Part model, mm, in its own coordinate system. Face numbers are marked on the shaded views. A direction names the side the tool comes from. Give positions to 0.01 mm unless a question says otherwise; leave off trailing zeros. Order: outer loops, then holes, each group sorted by start corner. A loop starts at its lowest first (then second) coordinate and runs counter-clockwise, first axis right, second up. Notation, with made-up numbers: (0.25, 69) - (23.25, 69) arc R28 cw to (23.25, 93) - close; hole circle Ø7 at (10.5, -18.5). An arc over 180 degrees is marked (long way). One line per item, written item: value.
```python
from build123d import *

# Parameters (mm, degrees)
F0_W     = 31.8262
F0_H     = 7.8232
F1_DEPTH = 9.6012
F3_R     = 2.4511
F4_DEPTH = 1.8288
F5_W     = 28.9814
F5_H     = 4.826
F6_DEPTH = 8.382
F7_R     = 1.4478
F8_DEPTH = 8.382


with BuildPart() as f1:
    # F0 (on Top) → F1 (new body)
    with BuildSketch(Plane.XY):
        Rectangle(F0_W, F0_H)
    extrude(amount=F1_DEPTH)

    # F3 (on face) → F4 (join)
    with BuildSketch(Plane.XY.offset(9.6012)):
        with Locations((11.9888, 0)):
            Circle(F3_R)
        with Locations((3.9116, 0)):
            Circle(F3_R)
        with Locations((-3.9116, 0)):
            Circle(F3_R)
        with Locations((-11.9888, 0)):
            Circle(F3_R)
    extrude(amount=F4_DEPTH)

    # F5 (on face) → F6 (cut)
    with BuildSketch(Plane(origin=(0, 0, 0), x_dir=(1, 0, 0), z_dir=(0, 0, -1))):
        Rectangle(F5_W, F5_H)
    extrude(amount=-F6_DEPTH, mode=Mode.SUBTRACT)

    # F7 (on face) → F8 (join)
    with BuildSketch(Plane(origin=(0, 0, 8.382), x_dir=(1, 0, 0), z_dir=(0, 0, -1))):
        with Locations((-8.1915, 0)):
            Circle(F7_R)
        Circle(F7_R)
        with Locations((8.1915, 0)):
            Circle(F7_R)
    extrude(amount=F8_DEPTH)


solid = f1.part
```
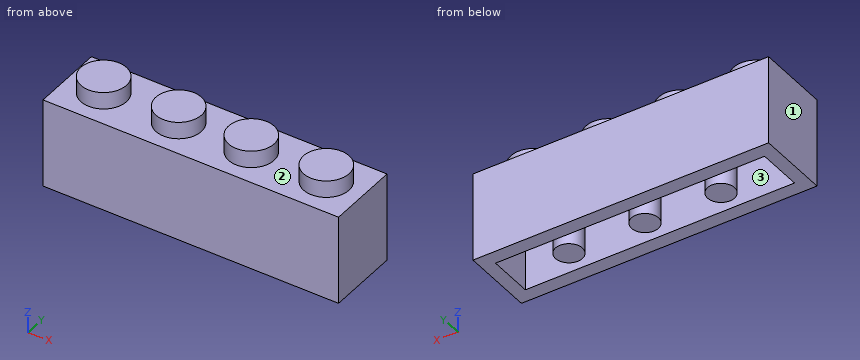
1) Which spindle directions (+Z, -Z, +X, -X, +Y, -Y) get a long thin tool onto all of the face, cutting with end or side? Do the marked faces 1, 2 and 3. Say none if no direction does.
Answer:
face 1: +Z, -Z, -X, +Y, -Y
face 2: +Z
face 3: -Z
2) Wall check: line 1 along X through (y, z) = (-1.5, 7.25); line 2 along Y through (x, z) = (-6.5, 3); line 3 along Y through (x, z) = (-0.5, 8). Give the ranges that are in metal, low to high. Write a range as [from, to].
Answer:
line 1: x = [-15.91, -14.49], [14.49, 15.91]
line 2: y = [-3.91, -2.41], [2.41, 3.91]
line 3: y = [-3.91, -2.41], [-1.36, 1.36], [2.41, 3.91]
3) Slice it at C-C on x = -13. Write the cut outline in (y, z).
Answer:
outline: (-3.91, 0) - (-2.41, 0) - (-2.41, 8.38) - (2.41, 8.38) - (2.41, 0) - (3.91, 0) - (3.91, 9.6) - (2.23, 9.6) - (2.23, 11.43) - (-2.23, 11.43) - (-2.23, 9.6) - (-3.91, 9.6) - close
4) Slice it at D-D on y = -1.75. Write the cut outline in (x, z).
Answer:
outline: (-15.91, 0) - (-14.49, 0) - (-14.49, 8.38) - (14.49, 8.38) - (14.49, 0) - (15.91, 0) - (15.91, 9.6) - (13.71, 9.6) - (13.71, 11.43) - (10.27, 11.43) - (10.27, 9.6) - (5.63, 9.6) - (5.63, 11.43) - (2.2, 11.43) - (2.2, 9.6) - (-2.2, 9.6) - (-2.2, 11.43) - (-5.63, 11.43) - (-5.63, 9.6) - (-10.27, 9.6) - (-10.27, 11.43) - (-13.71, 11.43) - (-13.71, 9.6) - (-15.91, 9.6) - close
5) Drop flat-ended pins along their axis: P1, Ø2.5, axis at x = -4, y = 1, coming from the -Z side; P2, Ø1, axis at x = -0.5, y = 2.5, coming from the -Z side. Give the stop position or say it passes through.
Answer:
P1: stops at z = 8.38
P2: stops at z = 0
6) Slice it at B-B on z = 10.5. Write the cut outline in (x, y), then the cut area to 3 significant figures.
Answer:
outline: circle Ø4.9 at (-11.99, 0); circle Ø4.9 at (-3.91, 0); circle Ø4.9 at (3.91, 0); circle Ø4.9 at (11.99, 0)
area: 75.5 mm2
7) Slice it at A-A on z = 6.5. Write the cut outline in (x, y).
Answer:
outline: (-15.91, -3.91) - (15.91, -3.91) - (15.91, 3.91) - (-15.91, 3.91) - close; circle Ø2.9 at (-8.19, 0); circle Ø2.9 at (0, 0); circle Ø2.9 at (8.19, 0); hole (-14.49, -2.41) - (14.49, -2.41) - (14.49, 2.41) - (-14.49, 2.41) - close
